Check sheet for the modelled part. Datum: model origin and axes. Units: mm. A direction names the side the tool comes from. Give positions to 0.01 mm unless a question says otherwise; leave off trailing zeros. Loops run counter-clockwise (first coordinate to the right, second up) from the corner with the lowest first, then second, coordinate; pieces in that order, holes last. Notation, with made-up numbers: M 4.25,75.5 L 11.25,75.5 A20 ccw 11.25,95.5 Z; hole C 31.5,-36.75 d9. An arc over 180 degrees is marked long. Use one line per item in the form item = value.
from build123d import *

# Parameters (mm, degrees)
SKETCH_1_R                   = 25
SKETCH_1_R_2                 = 21
EXTRUDE_1_DEPTH              = 10
EXTRUDE_START                = -4
SKETCH_1_5_R                 = 25
EXTRUDE_2_DEPTH              = 4
EXTRUDE_3_DEPTH              = 4
PATTERN_CIRCULAR_1_COUNT     = 6
HOLE_WIZARD_M3_2_D           = 3.4
HOLE_WIZARD_M3_2_CSINK_D     = 3.45
HOLE_WIZARD_M3_2_CSINK_ANGLE = 90


# Read off the part's stored shape, not the designer's step: M3 间隙孔1
with BuildPart() as part:
    # 草图1 → 拉伸-薄壁1 (new body)
    with BuildSketch(Plane(origin=(0, 0, 0), x_dir=(1, 0, 0), z_dir=(0, 1, 0))):
        Circle(SKETCH_1_R)
        Circle(SKETCH_1_R_2, mode=Mode.SUBTRACT)
    extrude(amount=EXTRUDE_1_DEPTH)

    # 草图1<5> → 凸台-拉伸2 (add)
    with BuildSketch(Plane(origin=(0, 0, 0), x_dir=(1, 0, 0), z_dir=(0, 1, 0)).offset(EXTRUDE_START)):
        with Locations(Location((0, 0, 0), (0, 0, 270))):
            Circle(SKETCH_1_5_R)
    extrude(amount=EXTRUDE_2_DEPTH)

    # 草图3 → 凸台-拉伸3 (add)
    with BuildSketch(Plane(origin=(0, 10, 0), x_dir=(1, 0, 0), z_dir=(0, 1, 0)).offset(EXTRUDE_START)):
        with BuildLine():
            ThreePointArc((-29.34, 4.5), (-33.84, 0), (-29.34, -4.5))
            Line((-29.34, -4.5), (-24.591665255, -4.5))
            ThreePointArc((-24.591665255, -4.5), (-25, 0), (-24.591665255, 4.5))
            Line((-24.591665255, 4.5), (-29.34, 4.5))
        make_face()
        with BuildLine():
            ThreePointArc((24.591665255, 4.5), (24.897707037, 2.259244191), (25, 0))
            ThreePointArc((25, 0), (24.897707037, -2.259244191), (24.591665255, -4.5))
            Line((24.591665255, -4.5), (29.34, -4.5))
            ThreePointArc((29.34, -4.5), (33.84, 0), (29.34, 4.5))
            Line((29.34, 4.5), (24.591665255, 4.5))
        make_face()
        with BuildLine():
            Line((-4.5, 29.34), (-4.5, 24.591665255))
            ThreePointArc((-4.5, 24.591665255), (0, 25), (4.5, 24.591665255))
            Line((4.5, 24.591665255), (4.5, 29.34))
            ThreePointArc((4.5, 29.34), (0, 33.84), (-4.5, 29.34))
        make_face()
        with BuildLine():
            ThreePointArc((4.5, -24.591665255), (0, -25), (-4.5, -24.591665255))
            Line((-4.5, -24.591665255), (-4.5, -29.34))
            ThreePointArc((-4.5, -29.34), (0, -33.84), (4.5, -29.34))
            Line((4.5, -29.34), (4.5, -24.591665255))
        make_face()
    extrude(amount=EXTRUDE_3_DEPTH)

    # M3 间隙孔1 outline → M3 间隙孔1 (revolve, cut)
    with BuildSketch(Plane(origin=(-13.5, 0, 0), x_dir=(1, 0, 0), z_dir=(0, 0, 1))):
        Polygon((1.7, -3.975), (1.7, 0), (0, 0), (0, -4), (1.725, -4), align=None)
    hole_wizard_m3_1 = revolve(axis=Axis((-13.5, 0, 0), (0, 1, 0)), mode=Mode.SUBTRACT)

    # 阵列(圆周)1: M3 间隙孔1 ×6 about axis
    pattern_circular_1_axis = Axis((0, 0, 0), (0, 1, 0))
    for i in range(1, PATTERN_CIRCULAR_1_COUNT):
        add(hole_wizard_m3_1.rotate(pattern_circular_1_axis, i * 360 / PATTERN_CIRCULAR_1_COUNT), mode=Mode.SUBTRACT)

    # M3 间隙孔2 (through all)
    with Locations(Plane(origin=(0, 6, 0), x_dir=(-1, 0, 0), z_dir=(0, -1, 0))):
        with Locations((0, 29.34), (29.34, 0), (0, -29.34), (-29.34, 0)):
            CounterSinkHole(HOLE_WIZARD_M3_2_D / 2, HOLE_WIZARD_M3_2_CSINK_D / 2, counter_sink_angle=HOLE_WIZARD_M3_2_CSINK_ANGLE)


solid = part.part
1) Release check for a two-part mould opening along Z. For faces 1 (the face through (0, 0, 0)), 2 (the face through (-27, 8, 4.5)), 3 (the face through (-33.84, 7.97, -0.1)) record: pulls with the +Z half, pulls with the -Z half, needs draft (parallel to the pull), parting line crosses it, or undercut.
Evaluation:
face_1 = undercut
face_2 = pulls with the +Z half
face_3 = parting line crosses it
2) Section check A-A (x = 0). Record the cut outline in (y, z) (3 decimals).
Evaluation:
outline = M -4,-25 L 6,-25 L 6,-27.615 L 6.025,-27.64 L 10,-27.64 L 10,-21 L 0,-21 L 0,21 L 10,21 L 10,27.64 L 6.025,27.64 L 6,27.615 L 6,25 L -4,25 Z; M 6,-33.84 L 10,-33.84 L 10,-31.04 L 6.025,-31.04 L 6,-31.065 Z; M 6,31.065 L 6.025,31.04 L 10,31.04 L 10,33.84 L 6,33.84 Z
3) Section check C-C (x = 13.5). Record the cut outline in (y, z) (3 decimals).
Evaluation:
outline = M -4,-21.042 L 10,-21.042 L 10,-16.086 L 0,-16.086 L 0,-1.7 L -3.975,-1.7 L -4,-1.725 Z; M -4,1.725 L -3.975,1.7 L 0,1.7 L 0,16.086 L 10,16.086 L 10,21.042 L -4,21.042 Z
4) Scan lines: line 1 (Z direction, x = 0, y = 9); line 2 (Z direction, x = 29.34, y = 9); line 3 (Z direction, x = -6.75, y = -3.05). Record each from-to range of solid material in increasing order.
Evaluation:
line_1 = -33.84 to -31.04, -27.64 to -21, 21 to 27.64, 31.04 to 33.84
line_2 = -4.5 to -1.7, 1.7 to 4.5
line_3 = -24.07 to -13.39, -9.99 to 9.99, 13.39 to 24.07
5) Set-up check for faces 4 (the face through (27, 8, 4.5)), 5 (the face through (4.5, 8, -27)), 6 (the face through (0.1, 7.97, -33.84)): record each of +Z, -Z, +X, -X, +Y, -Y from which the full face is reachable in a straight line by a thin tool's end or side.
Evaluation:
face_4 = +Z, +X, +Y, -Y
face_5 = -Z, +X, +Y, -Y
face_6 = -Z, +Y, -Y
6) Section check B-B (z = 0). State how many separate pieces and enclosed holes the cut face has, then the cut area to 3 significant figures.
Evaluation:
separate_pieces = 5
enclosed_holes = 0
area = 296 mm^2
7) Depth check by flat-ended pin: pin 1 Ø4 at (x, z) = (6.75, 11.69) entering from +Y; pin 2 Ø4 at (y, z) = (7.5, -19.5) entering from -X; pin 3 Ø5 at (x, y) = (-24, -0.5) entering from -Z. Enter the tip coordinate at first touch or a pass-through.
Evaluation:
pin_1 = 0
pin_2 = -17.85
pin_3 = -12.76
